Drawing for the job (mm, zero at the part's lowest x, y, z). A direction names the side the tool comes from. Coordinates: 2 decimals unless noted, no trailing zeros. Loops run counter-clockwise (first coordinate to the right, second up) from the corner with the lowest first, then second, coordinate; pieces in that order, holes last. Notation, with made-up numbers: (-24, 5) -> (-18, 5) arc R30 ccw to (-18, 36) -> close; hole circle Ø4 at (-12, 0.25). An arc over 180 degrees is marked (long way). Write item = value, one per line. Start each with the question number.
(1) Tool access for the marked faces 1 and 2: list every direction of +Z, -Z, +X, -X, +Y, -Y with a clear straight run to the whole face (end or side of a thin tool).
(2) Drill centre lines: line 1 (Y direction, x = 21.5, z = 35); line 2 (Z direction, x = 3.5, y = 11) (1 decimal); line 3 (X direction, y = 7, z = 18.5). Where is each one in solid material? Low to high. Write a range as from..to.
(3) Flat gauge pins, fed straight in: P1, Ø1.5, axis at x = 19.05, z = 36.17, coming from the -Y side; P2, Ø6, axis at x = 29, y = 2.5, coming from the -Z side; P3, Ø4, axis at x = 21, y = 7, coming from the +Z side; P4, Ø2, axis at y = 2, z = 5, coming from the -X side. Where does each tip first touch, or does it go through?
(4) Band-saw the part on D-D (x = 13). Write the cut outline in (y, z), and give its area (3 significant figures).
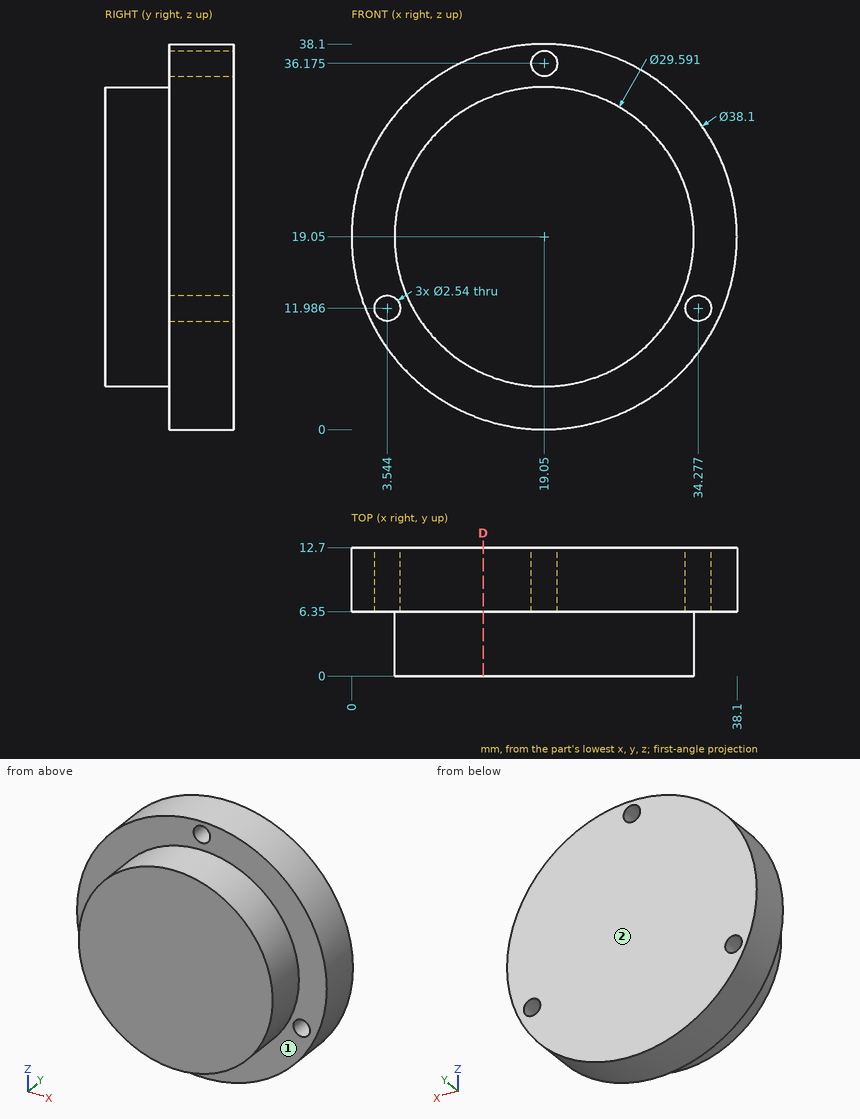
Findings below:
q1.face_1 = -Y
q1.face_2 = +Z, -Z, +X, -X, +Y
q2.line_1 = 6.35..12.7
q2.line_2 = 8..10.7, 13.3..30.1
q2.line_3 = 0.01..38.09
q3.P1 = through
q3.P2 = 5.99
q3.P3 = 38.1
q3.P4 = 12.08
q4.outline = (0, 5.55) -> (6.35, 5.55) -> (6.35, 0.99) -> (12.7, 0.99) -> (12.7, 37.11) -> (6.35, 37.11) -> (6.35, 32.55) -> (0, 32.55) -> close
q4.area = 401 mm²
